The drawing under review shows one solid part. Ordinate dimensions are in mm from its lowest x, y, z. A direction names the side the tool comes from. Coordinates: 2 decimals unless noted, no trailing zeros. Write each loop counter-clockwise with the first axis right and the second up, starting at its lowest first coordinate (ties: lowest second). Pieces come first, ordered by that corner, then holes.
1) Machinability: for the marked faces 5 and 6, which of the approach directions +Z, -Z, +X, -X, +Y, -Y give a long, thin tool a straight path to every point of the face, cutting with its end or side? Answer none if there is none.
2) Mouldability with a two-part tool opening along Y and no side actions: class the marked faces 1, 2, 3 and 4 as released by +Y, released by -Y, zero draft, split by the parting line, or undercut.
3) Add section D-D, the plane y = 67.5. State the section outline as (x, z) points, then the cut area to 3 significant figures.
4) Add section A-A, the plane x = 13.5. State the section outline as (y, z) points.
5) Add section C-C, the plane x = 71.5. State the section outline as (y, z) points.
6) Add section B-B, the plane z = 4.5. State the section outline as (x, y) points, then the cut area to 3 significant figures.
7) For line 1 (Y direction, x = 63.5, z = 12); line 2 (X direction, y = 5.5, z = 10); line 3 (Z direction, x = 70, y = 92), list the stretches that pass through material, from the lowest coordinate up.
8) For P1, Ø6, axis at y = 47.5, z = 8.5, coming from the +X side; P2, Ø4, axis at x = 14, z = 5, coming from the -Y side, all flat-tipped, find the tip position at first contact; note any pin that passes through.
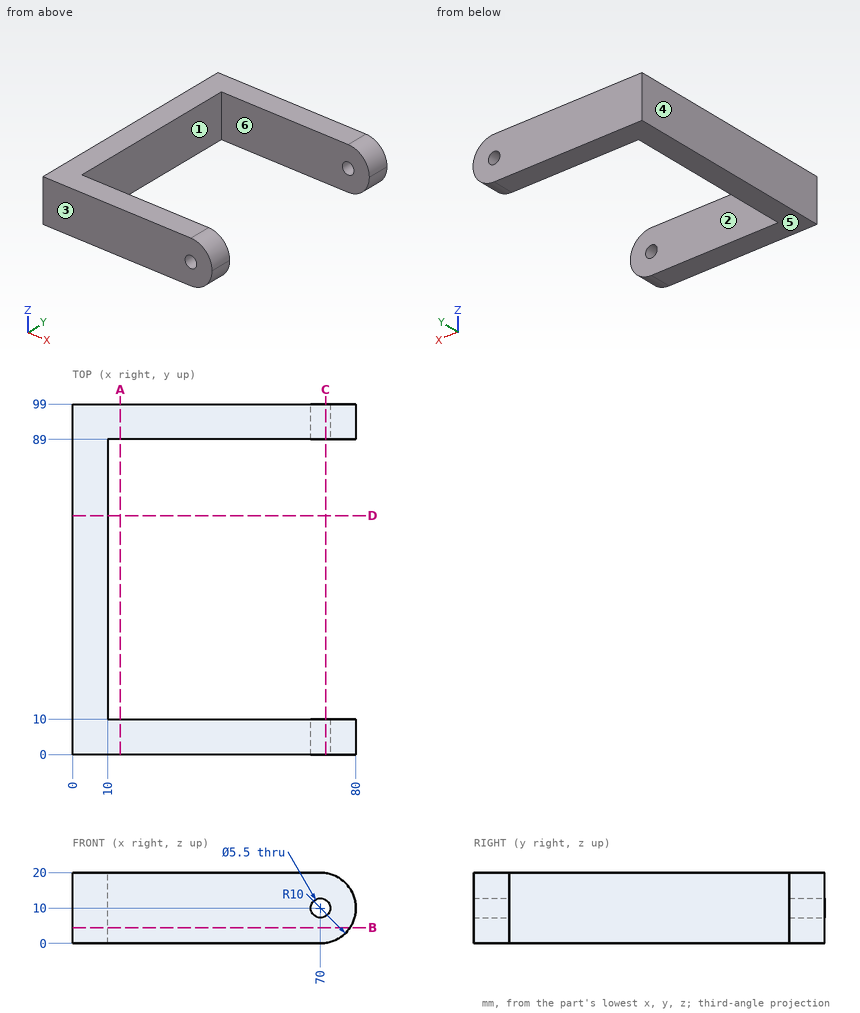
Geometry results:
1. face 5: -Z, +X, -X, +Y, -Y
1. face 6: +Z, -Z, +X
2. face 1: undercut
2. face 2: undercut
2. face 3: released by -Y
2. face 4: zero draft
3. outline: (0, 0) - (10, 0) - (10, 20) - (0, 20) - close
3. area: 200 mm2
4. outline: (0, 0) - (10, 0) - (10, 20) - (0, 20) - close; (89, 0) - (99, 0) - (99, 20) - (89, 20) - close
5. outline: (0, 0.11) - (10, 0.11) - (10, 7.7) - (0, 7.7) - close; (0, 12.3) - (10, 12.3) - (10, 19.89) - (0, 19.89) - close; (89, 0.11) - (99, 0.11) - (99, 7.7) - (89, 7.7) - close; (89, 12.3) - (99, 12.3) - (99, 19.89) - (89, 19.89) - close
6. outline: (0, 0) - (78.35, 0) - (78.35, 10) - (10, 10) - (10, 89) - (78.35, 89) - (78.35, 99) - (0, 99) - close
6. area: 2,360 mm2
7. line 1: y = 0 to 10, 89 to 99
7. line 2: x = 0 to 67.25, 72.75 to 80
7. line 3: z = 0 to 7.25, 12.75 to 20
8. P1: stops at x = 10
8. P2: stops at y = 0
